Geometry: final body of the model. Coordinates: model frame, mm. Face numbers are marked on the shaded views. A direction names the side the tool comes from. Coordinates: 2 decimals unless noted, no trailing zeros. Write each loop counter-clockwise with the first axis right and the second up, starting at its lowest first coordinate (ties: lowest second). Pieces come first, ordered by that corner, then holes. Notation, with made-up numbers: (28, 28.25) - (45, 28.25) arc R24 cw to (45, 51.25) - close; hole circle Ø8 at (-5.5, 89.5). An arc over 180 degrees is marked (long way). Answer as a JSON object with one key per item and string values. Group by question number.
Item 1: Set-up query: the marked faces 1 and 2. Return all of +Z, -Z, +X, -X, +Y, -Y with unobstructed straight access to the full face (end or side cutting, diameter ignored); none if empty.
Item 2: Line query: line 1 along Y through (x, z) = (29, 0.65); line 2 along X through (y, z) = (21, 2.9); line 3 along X through (y, z) = (7, 2.1). Output: solid intervals per line, ascending. Write a range as from..to.
Item 3: Mould query, pull axis X, two halves, no side actions, for the marked faces 3, 4 and 5. Classes: pulls with the +X half, pulls with the -X half, needs draft (parallel to the pull), parting line crosses it, or undercut.
Item 4: Section C-C on y = 14. Return loops of the section in (x, z).
Item 5: First-contact query: pin 1 Ø0.6 at (y, z) = (35.5, 2) entering from -X. Flat tip, straight axial feed; report the tip coordinate or a pass-through.
Item 6: Section D-D on x = 16. Return loops of the section in (y, z), and give its area (3 significant figures).
Item 7: Section B-B on z = 3.2. Return loops of the section in (x, y), and give its area (3 significant figures).
Item 8: Section A-A on x = 24.5. Return loops of the section in (y, z).
Autodesk Inventor part; units mm, degrees
ref_plane "YZ Plane" through (0, 0, 0) normal (1, 0, 0) x (0, 1, 0)
ref_plane "XZ Plane" through (0, 0, 0) normal (0, 1, 0) x (-1, 0, 0)
ref_plane "XY Plane" through (0, 0, 0) normal (0, 0, 1) x (1, 0, 0)
sketch "Esquisse1" plane through (0, 0, 0) normal (0, 0, 1) x (1, 0, 0)
  line L0 (0, 0) -> (0, 32.5)
  line L1 (0, 0) -> (58.5, 0)
  line L2 (58.5, 0) -> (58.5, 42.9)
  line L3 (58.5, 42.9) -> (21, 42.9)
  line L4 (0, 32.5) -> (21, 42.9)
  line L5 (58.5, 42.9) -> (0, 42.9) construction
  line L6 (0, 42.9) -> (0, 0) construction
  line L7 (0, 42.9) -> (58.5, 0) construction
  line L8 (58.5, 42.9) -> (0, 0) construction
  dimension "d0" = 32.5
  dimension "d1" = 58.5
  dimension "d2" = 42.9
  dimension "d3" = 37.5
extrude "Extrusion1" add sketch "Esquisse1" along normal blind 5
sketch "Esquisse2" plane through (0, 0, 5) normal (0, 0, 1) x (1, 0, 0)
  line L0 (23.25, 32.95) -> (35.25, 32.95)
  line L1 (35.25, 32.95) -> (35.25, 9.95)
  line L2 (35.25, 9.95) -> (23.25, 9.95)
  line L3 (23.25, 9.95) -> (23.25, 32.95)
  line L4 (0, 32.5) -> (0, 0)
  line L5 (58.5, 42.9) -> (21, 42.9)
  line L6 (28.25, 36.45) -> (30.25, 36.45)
  line L7 (30.25, 36.45) -> (30.25, 34.45)
  line L8 (30.25, 34.45) -> (28.25, 34.45)
  line L9 (28.25, 34.45) -> (28.25, 36.45)
  line L10 (28.25, 8.45) -> (30.25, 8.45)
  line L11 (30.25, 8.45) -> (30.25, 6.45)
  line L12 (30.25, 6.45) -> (28.25, 6.45)
  line L13 (28.25, 6.45) -> (28.25, 8.45)
  dimension "d6" = 23
  dimension "d7" = 12
  dimension "d8" = 23.25
  dimension "d9" = 9.95
  dimension "d10" = 2
  dimension "d11" = 2
  dimension "d12" = 2
  dimension "d13" = 2
  dimension "d14" = 1.5
  dimension "d15" = 1.5
  dimension "d16" = 5
  dimension "d17" = 5
extrude "Extrusion2" cut sketch "Esquisse2" against normal blind 5
properties part number "BackHand" material "Plastique ABS"
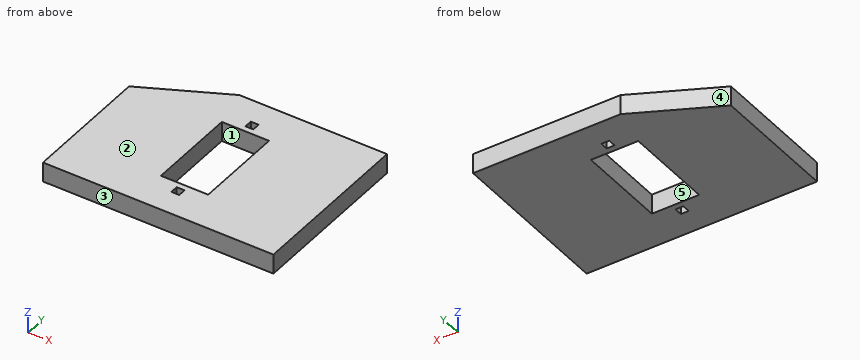
Checks:
{
 "1": {"face 1": "+Z, -Z", "face 2": "+Z, +X, -X, +Y, -Y"},
 "2": {"line 1": "0..6.45, 8.45..9.95, 32.95..34.45, 36.45..42.9", "line 2": "0..23.25, 35.25..58.5", "line 3": "0..28.25, 30.25..58.5"},
 "3": {"face 3": "needs draft", "face 4": "pulls with the -X half", "face 5": "undercut"},
 "4": {"outline": "(0, 0) - (23.25, 0) - (23.25, 5) - (0, 5) - close; (35.25, 0) - (58.5, 0) - (58.5, 5) - (35.25, 5) - close"},
 "5": {"pin 1": "x = 5.45"},
 "6": {"outline": "(0, 0) - (40.42, 0) - (40.42, 5) - (0, 5) - close", "area": "202 mm^2"},
 "7": {"outline": "(0, 0) - (58.5, 0) - (58.5, 42.9) - (21, 42.9) - (0, 32.5) - close; hole (23.25, 9.95) - (35.25, 9.95) - (35.25, 32.95) - (23.25, 32.95) - close; hole (28.25, 6.45) - (30.25, 6.45) - (30.25, 8.45) - (28.25, 8.45) - close; hole (28.25, 34.45) - (30.25, 34.45) - (30.25, 36.45) - (28.25, 36.45) - close", "area": "2,120 mm^2"},
 "8": {"outline": "(0, 0) - (9.95, 0) - (9.95, 5) - (0, 5) - close; (32.95, 0) - (42.9, 0) - (42.9, 5) - (32.95, 5) - close"}
}
